```python
from build123d import *

# Parameters (mm, degrees)
F0_R     = 31
F0_R_2   = 3
F1_DEPTH = 40
F3_DEPTH = 80
F4_R     = 0.75
F5_DEPTH = 15
F6_SIZE  = 2


with BuildPart() as f1:
    # F0 (on Front) → F1 (new body)
    with BuildSketch(Plane.XZ):
        Circle(F0_R)
        with Locations((-17.960512, -17.960512)):
            Circle(F0_R_2, mode=Mode.SUBTRACT)
        with Locations((17.960512, -17.960512)):
            Circle(F0_R_2, mode=Mode.SUBTRACT)
        with Locations((-17.960512, 17.960512)):
            Circle(F0_R_2, mode=Mode.SUBTRACT)
        with Locations((17.960512, 17.960512)):
            Circle(F0_R_2, mode=Mode.SUBTRACT)
    extrude(amount=F1_DEPTH)

    # F2 (on face) → F3 (join)
    with BuildSketch(Plane.XZ.offset(40)):
        with BuildLine():
            ThreePointArc((19.4, 0), (7.424059, 17.923263), (-13.717872, 13.717872))
            ThreePointArc((-13.717872, 13.717872), (-7.424059, -17.923263), (19.4, 0))
        make_face()
    extrude(amount=F3_DEPTH)

    # F4 (on face) → F5 (cut)
    with BuildSketch(Plane.XZ.offset(120)):
        with Locations((-6, 0)):
            Circle(F4_R)
        with Locations((-6, -8)):
            Circle(F4_R)
    extrude(amount=-F5_DEPTH, mode=Mode.SUBTRACT)

    # F6
    f6_edges = [f1.edges().sort_by_distance(p)[0] for p in [
        (-19.4, -120, 0),
        (-31, -40, 0),
    ]]
    chamfer(f6_edges, length=F6_SIZE)


solid = f1.part
```
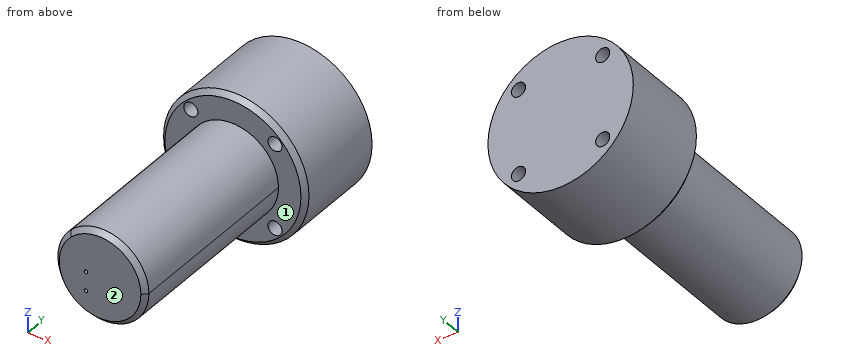
Can you work these out from the model? Positions are in its coordinate system, mm. Face numbers are marked on the shaded views. A direction names the side the tool comes from. Give positions to 0.01 mm unless a question says otherwise; leave off trailing zeros. Order: outer loops, then holes, each group sorted by start corner. A loop starts at its lowest first (then second) coordinate and runs counter-clockwise, first axis right, second up. Notation, with made-up numbers: M 63,40.25 L 100,40.25 A12 cw 100,53.25 Z; hole C 48.25,24 d5. An arc over 180 degrees is marked long. Write item = value, one per line. Start each with the question number.
Q1. I need wall thicknesses on probe 1 along Z at (x, y) = (-6, -113.75); probe 2 along X at (y, z) = (-23, -20.5); probe 3 along Y at (x, z) = (-23.5, -13). Which ranges of each line are inside material? Lowest first, please. Write a range as [from, to].
Q2. Will these pins go through, and if not, where does the flat tip stop? pin 1 Ø1.5 at (x, z) = (-21.5, -11.5) entering from +Y; pin 2 Ø4 at (x, y) = (-22.5, -25) entering from -Z; pin 3 Ø5 at (x, y) = (14, -18.5) entering from +Z; pin 4 Ø5 at (x, y) = (1, -33.5) entering from +Z.
Q3. Suppose I cut it at B-B (y = -20). Write out the boundary of the cut face in (x, z).
Q4. Suppose I cut it at A-A (y = -92). Write out the boundary of the cut face in (x, z), plus the area to 3 significant figures.
Q5. For the marked faces 1 and 2, which set-ups out of +Z, -Z, +X, -X, +Y, -Y let a thin tool reach every point of the face, with its end or its side?
Check result:
q1.probe_1 = [-18.45, -8.75], [-7.25, -0.75], [0.75, 18.45]
q1.probe_2 = [-23.25, -19.56], [-16.36, 16.36], [19.56, 23.25]
q1.probe_3 = [-40, 0]
q2.pin_1 = 0
q2.pin_2 = -23.25
q2.pin_3 = 28.79
q2.pin_4 = 31
q3.outline = C 0,0 d62; hole C -17.96,-17.96 d6; hole C -17.96,17.96 d6; hole C 17.96,-17.96 d6; hole C 17.96,17.96 d6
q4.outline = C 0,0 d38.8
q4.area = 1,180 mm2
q5.face_1 = -Y
q5.face_2 = +Z, -Z, +X, -X, -Y
